Autodesk Inventor part; units mm, degrees
ref_plane "YZ Plane" through (0, 0, 0) normal (1, 0, 0) x (0, 1, 0)
ref_plane "XZ Plane" through (0, 0, 0) normal (0, 1, 0) x (-1, 0, 0)
ref_plane "XY Plane" through (0, 0, 0) normal (0, 0, 1) x (1, 0, 0)
sketch "Sketch1" plane through (0, 0, 0) normal (0, 1, 0) x (-1, 0, 0)
  line L0 (-7.5, 7.5) -> (7.5, 7.5)
  line L1 (7.5, 7.5) -> (7.5, -7.5)
  line L2 (7.5, -7.5) -> (-7.5, -7.5)
  line L3 (-7.5, -7.5) -> (-7.5, 7.5)
  line L4 (-7.5, 7.5) -> (7.5, -7.5) construction
  line L5 (7.5, 7.5) -> (-7.5, -7.5) construction
  point P0 (0, 0)
  dimension "d0" = 15
  dimension "d1" = 15
extrude "Extrusion1" add sketch "Sketch1" along normal blind 2
sketch "Sketch2" plane through (0, 2, 0) normal (0, 1, 0) x (1, 0, 0)
  line L0 (7.5, 7.5) -> (-7.5, 7.5) construction
  line L1 (-7.5, 7.5) -> (-7.5, -7.5) construction
  line L2 (-7.5, -7.5) -> (7.5, -7.5) construction
  line L3 (7.5, -7.5) -> (7.5, 7.5) construction
  line L4 (-7.5, 7.5) -> (-7.5, -7.5)
  line L5 (-7.5, 0) -> (-0.5, 0)
  line L6 (-0.5, 0) -> (-0.5, 4)
  line L7 (-0.5, 4) -> (-7.5, 4)
  line L8 (-7.5, 4) -> (-7.5, 0)
  line L9 (-7.5, 0) -> (-0.5, 0) construction
  line L10 (-7.5, 0) -> (-0.5, 0)
  line L11 (-0.5, 0) -> (-0.5, -4)
  line L12 (-0.5, -4) -> (-7.5, -4)
  line L13 (-7.5, -4) -> (-7.5, 0)
  point P0 (0, 0)
  point P1 (-7.5, 4)
  dimension "d4" = 7
  dimension "d5" = 0
  dimension "d6" = 4
  dimension "d7" = 4
extrude "Extrusion2" add sketch "Sketch2" along normal blind 3
sketch "Sketch3" plane through (0, 2, 0) normal (0, 1, 0) x (1, 0, 0)
  line L0 (-0.5, 4) -> (-0.5, -4) construction
  line L1 (7.5, 7.5) -> (-7.5, 7.5) construction
  line L2 (7.5, 4.75) -> (2.5, 4.75) construction
  circle A0 centre (2.5, 4.75) radius 1.75
  line L3 (7.5, -7.5) -> (7.5, 7.5) construction
  line L4 (0, 0) -> (7.5, 0) construction
  line L5 (7.5, -7.5) -> (7.5, 7.5) construction
  circle A1 centre (2.5, -4.75) radius 1.75
  dimension "d10" = 5
  dimension "d11" = 3.5
  dimension "d12" = 2.75
extrude "Extrusion3" cut sketch "Sketch3" against normal through all
equation "\"d7\" = d6"
properties part number "Charger_Port"
Work out the finished part from the listing and answer in its coordinate system (mm). A direction names the side the tool comes from. Give positions to 0.01 mm unless a question says otherwise; leave off trailing zeros. Loops run counter-clockwise (first coordinate to the right, second up) from the corner with the lowest first, then second, coordinate; pieces in that order, holes last. Notation, with made-up numbers: M 78.5,69 L 136.5,69 A13 ccw 136.5,90 Z; hole C 54.25,-4 d9. An arc over 180 degrees is marked long. One line per item, written item: value. Start each with the question number.
1. Find section D-D (z = 2). Give the vertices of the cut face in (x, y).
2. Which of the six approach directions +Z, -Z, +X, -X, +Y, -Y give full straight-line access (tool end or side, diameter ignored) to faces 5 (the face through (-7.5, 2, 0)), 6 (the face through (-4, 3, 4)), 7 (the face through (0, 1, 7.5)), 8 (the face through (-4, 3, -4)), 9 (the face through (-0.5, 3, 0))?
3. Find section B-B (z = -4.75). Give the vertices of the cut face in (x, y), and give its area (3 significant figures).
4. Determine the mould class of faces 1 (the face through (0, 1, -7.5)), 2 (the face through (4.117, 1.014, 5.42)), 3 (the face through (3.31, 1.01, -3.2)), 4 (the face through (-4, 5, 0)) for opening direction Z: released by +Z, released by -Z, zero draft, split by the parting line, or undercut.
5. Find the intervals of material crossed by probe 1 along Z at (x, y) = (2.5, 0.5); probe 2 along X at (y, z) = (0.45, 4.75); probe 3 along Y at (x, z) = (-1, -4.25), in increasing order.
6. Each of these flat-tipped pins is pushed along its axis until it touches: P1, Ø0.9, axis at x = -4.5, y = 3, coming from the +Z side; P2, Ø1.5, axis at y = 3.5, z = 1.5, coming from the +X side; P3, Ø0.9, axis at x = -4, y = 3, coming from the -Z side. Where does it stop, or does it pass through?
7. Find section C-C (x = -1.25). Give the vertices of the cut face in (y, z), and give its area (3 significant figures).
8. Find section A-A (x = 2.5). Give the vertices of the cut face in (y, z).
Reported:
1. outline: M -7.5,0 L 7.5,0 L 7.5,2 L -0.5,2 L -0.5,5 L -7.5,5 Z
2. face 5: +Z, -Z, -X, +Y, -Y
2. face 6: +Z, +X, -X, +Y
2. face 7: +Z, +X, -X, +Y, -Y
2. face 8: -Z, +X, -X, +Y
2. face 9: +Z, -Z, +X, +Y
3. outline: M -7.5,0 L 0.75,0 L 0.75,2 L -7.5,2 Z; M 4.25,0 L 7.5,0 L 7.5,2 L 4.25,2 Z
3. area: 23.0 mm²
4. face 1: released by -Z
4. face 2: undercut
4. face 3: undercut
4. face 4: zero draft
5. probe 1: z = -7.5 to -6.5, -3 to 3, 6.5 to 7.5
5. probe 2: x = -7.5 to 0.75, 4.25 to 7.5
5. probe 3: y = 0 to 2
6. P1: stops at z = 4
6. P2: stops at x = -0.5
6. P3: stops at z = -4
7. outline: M 0,-7.5 L 2,-7.5 L 2,-4 L 5,-4 L 5,4 L 2,4 L 2,7.5 L 0,7.5 Z
7. area: 54.0 mm²
8. outline: M 0,-7.5 L 2,-7.5 L 2,-6.5 L 0,-6.5 Z; M 0,-3 L 2,-3 L 2,3 L 0,3 Z; M 0,6.5 L 2,6.5 L 2,7.5 L 0,7.5 Z
